Verification items for the finished model (mm, model axes). Face numbers are marked on the shaded views. A direction names the side the tool comes from. Coordinates: 2 decimals unless noted, no trailing zeros. Loops run counter-clockwise (first coordinate to the right, second up) from the corner with the lowest first, then second, coordinate; pieces in that order, holes last. Notation, with made-up numbers: (58, 43.25) - (95, 43.25) arc R26 ccw to (95, 69.25) - close; hole circle Ø9 at (31.5, -14.75). An arc over 180 degrees is marked (long way). One line per item, written item: value. Start each with the question number.
(1) Thickness scan on probe 1 along X at (y, z) = (-9.75, 0); probe 2 along Z at (x, y) = (-2, 0); probe 3 along Z at (x, y) = (7, 0). Record the ranges inside material, lowest first. Write a range as [from, to].
(2) Section check B-B (y = 0). Record the boundary of the cut face in (x, z), plus the area to 3 significant figures.
(3) Gauge pin test, flat ends, axial feed: P1, Ø2, axis at x = 33.5, y = -7.5, coming from the -Z side; P2, Ø1, axis at x = 39.5, y = 2, coming from the +Z side; P3, Ø1.5, axis at x = 23.5, y = 9, coming from the -Z side; P4, Ø2, axis at x = 82.9, z = 0, coming from the -Y side. Record the tip position at first contact, or that the pin passes through.
(4) Section check C-C (x = 82.9). Record the boundary of the cut face in (y, z), plus the area to 3 significant figures.
(5) Draft check along Z on the marked faces 1 and 2. Enter one of: +Z half, -Z half, draft (parallel to the pull), parting line (faces both ways), or undercut.
(6) Section check A-A (z = 0). Record the boundary of the cut face in (x, y), plus the area to 3 significant figures.
(7) Set-up check for the marked faces 3 and 4: record each of +Z, -Z, +X, -X, +Y, -Y from which the full face is reachable in a straight line by a thin tool's end or side.
(8) Section check D-D (x = 47.5). Record the boundary of the cut face in (y, z), plus the area to 3 significant figures.
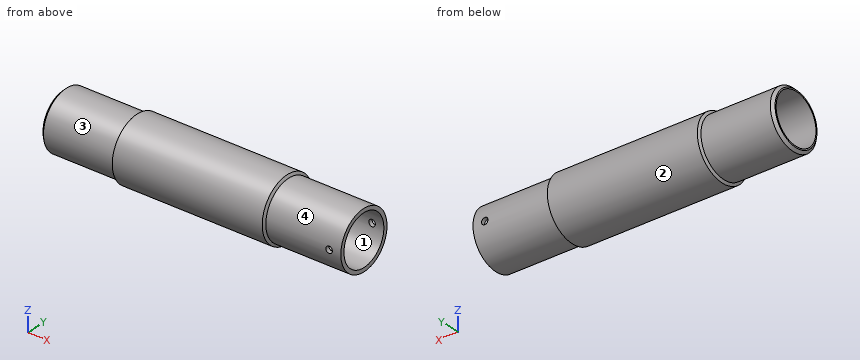
Autodesk Inventor part; units mm, degrees
ref_plane "YZ Plane" through (0, 0, 0) normal (1, 0, 0) x (0, 1, 0)
ref_plane "XZ Plane" through (0, 0, 0) normal (0, 1, 0) x (-1, 0, 0)
ref_plane "XY Plane" through (0, 0, 0) normal (0, 0, 1) x (1, 0, 0)
sketch "Profile" plane through (0, 0, 0) normal (0, 0, 1) x (1, 0, 0)
  line L0 (-27.6, 0) -> (-27.6, 11)
  line L1 (-27.6, 11) -> (0, 11)
  line L2 (0, 11) -> (0.5774, 12)
  line L3 (0.5774, 12) -> (58.0774, 12)
  line L4 (58.0774, 12) -> (58.6547, 11)
  line L5 (58.6547, 11) -> (87.4, 11)
  line L6 (87.4, 11) -> (87.4, 0)
  line L7 (-27.6, 0) -> (0, 0)
  line L8 (0, 0) -> (0, 9)
  line L9 (0, 9) -> (79.4, 9)
  line L10 (79.4, 9) -> (79.4, 0)
  line L11 (79.4, 0) -> (87.4, 0)
  line L12 (-50.6, 0) -> (110.4, 0) construction
  line L13 (0, 11) -> (0, 9) construction
  dimension "BodyLength" = 115
  dimension "d1" = 11
  dimension "d3" = 120
  dimension "d4" = 120
  dimension "d5" = 57.5
  dimension "d6" = 27.6
  dimension "d16" = 8
  dimension "d29" = 1
  dimension "d30" = 9
revolve "ProfileRevolveFeature" add sketch "Profile" angle 360 about axis through (-10, 0, 0) along (1, 0, 0)
sketch "InsideHole" plane through (-27.6, 0, 0) normal (-1, 0, 0) x (0, 0, 1)
  circle A0 centre (0, 0) radius 9 construction
hole "InsideHoleFeature" at (-27.6, 0, 0) direction (1, 0, 0) diameter 19 end through all
chamfer "EndChamferFeature" distance 1 angle 45 1 edges at (-27.6, -11, 0)
sketch "CapMountHole" plane through (0, 0, 0) normal (0, 1, 0) x (-1, 0, 0)
  line L0 (-87.4, 11) -> (-87.4, -11) construction
  line L1 (13.68, 0) -> (-82.08, 0) construction
  circle A0 centre (-82.9, 0) radius 1.25
  point P0 (0, 0)
  dimension "d31" = 4.5
  dimension "d39" = 2.5
extrude "CapMountHoleFeature" cut sketch "CapMountHole" along normal through all both and the other way through all
equation "\"d5\" = 0.5 * BodyLength"
equation "\"d6\" = 0.24 * BodyLength"
properties part number "BackPair1PistonBody"
Responses:
1. probe 1: x = [-27.6, 81.65], [84.15, 87.4]
1. probe 2: z = [-11, -9.5], [9.5, 11]
1. probe 3: z = [-12, -9.5], [9.5, 12]
2. outline: (-27.6, -10) - (-26.6, -11) - (0, -11) - (0.58, -12) - (58.08, -12) - (58.65, -11) - (87.4, -11) - (87.4, -9.5) - (-27.6, -9.5) - close; (-27.6, 9.5) - (87.4, 9.5) - (87.4, 11) - (58.65, 11) - (58.08, 12) - (0.58, 12) - (0, 11) - (-26.6, 11) - (-27.6, 10) - close
2. area: 460 mm²
3. P1: stops at z = -10.09
3. P2: stops at z = 11.91
3. P3: stops at z = -8.71
3. P4: passes through
4. outline: (-10.93, -1.25) arc R11 ccw to (10.93, -1.25) - (9.42, -1.25) arc R9.5 cw to (-9.42, -1.25) - close; (-10.93, 1.25) - (-9.42, 1.25) arc R9.5 cw to (9.42, 1.25) - (10.93, 1.25) arc R11 ccw to start
4. area: 89.1 mm²
5. face 1: undercut
5. face 2: parting line
6. outline: (-27.6, -10) - (-26.6, -11) - (0, -11) - (0.58, -12) - (58.08, -12) - (58.65, -11) - (81.65, -11) - (81.65, -9.5) - (-27.6, -9.5) - close; (-27.6, 9.5) - (81.65, 9.5) - (81.65, 11) - (58.65, 11) - (58.08, 12) - (0.58, 12) - (0, 11) - (-26.6, 11) - (-27.6, 10) - close; (84.15, -11) - (87.4, -11) - (87.4, -9.5) - (84.15, -9.5) - close; (84.15, 9.5) - (87.4, 9.5) - (87.4, 11) - (84.15, 11) - close
6. area: 453 mm²
7. face 3: -X
7. face 4: +X
8. outline: circle Ø24 at (0, 0); hole circle Ø19 at (0, 0)
8. area: 169 mm²
